from build123d import *

# Parameters (mm, degrees)
ESQUISSE1_R             = 25.4
BOSS_EXTRU_1_DEPTH      = 12.7
ESQUISSE2_R             = 1.3
ENL_V_MAT_EXTRU_1_DEPTH = 12.7


with BuildPart() as part:
    # Esquisse1 → Boss.-Extru.1 (new body)
    with BuildSketch(Plane.XY):
        Circle(ESQUISSE1_R)
    extrude(amount=BOSS_EXTRU_1_DEPTH)

    # Esquisse2 → Enlèv. mat.-Extru.1 (cut)
    with BuildSketch(Plane(origin=(0, 0, 0), x_dir=(-1, 0, 0), z_dir=(0, 0, -1))):
        Circle(ESQUISSE2_R)
        with Locations((0, 4.5)):
            Circle(ESQUISSE2_R)
        with Locations((0, 9)):
            Circle(ESQUISSE2_R)
        with Locations((0, 13.5)):
            Circle(ESQUISSE2_R)
        with Locations((0, 18)):
            Circle(ESQUISSE2_R)
        with Locations((3.897114317, 2.25)):
            Circle(ESQUISSE2_R)
        with Locations((3.897114317, -2.25)):
            Circle(ESQUISSE2_R)
        with Locations((0, -4.5)):
            Circle(ESQUISSE2_R)
        with Locations((-3.897114317, -2.25)):
            Circle(ESQUISSE2_R)
        with Locations((-3.897114317, 2.25)):
            Circle(ESQUISSE2_R)
        with Locations((4.5, 7.794228634)):
            Circle(ESQUISSE2_R)
        with Locations((7.794228634, 4.5)):
            Circle(ESQUISSE2_R)
        with Locations((9, 0)):
            Circle(ESQUISSE2_R)
        with Locations((7.794228634, -4.5)):
            Circle(ESQUISSE2_R)
        with Locations((4.5, -7.794228634)):
            Circle(ESQUISSE2_R)
        with Locations((0, -9)):
            Circle(ESQUISSE2_R)
        with Locations((-4.5, -7.794228634)):
            Circle(ESQUISSE2_R)
        with Locations((-7.794228634, -4.5)):
            Circle(ESQUISSE2_R)
        with Locations((-9, 0)):
            Circle(ESQUISSE2_R)
        with Locations((-7.794228634, 4.5)):
            Circle(ESQUISSE2_R)
        with Locations((-4.5, 7.794228634)):
            Circle(ESQUISSE2_R)
        with Locations((4.617271935, 12.685850381)):
            Circle(ESQUISSE2_R)
        with Locations((8.677632731, 10.341599982)):
            Circle(ESQUISSE2_R)
        with Locations((11.691342951, 6.75)):
            Circle(ESQUISSE2_R)
        with Locations((13.294904666, 2.344250399)):
            Circle(ESQUISSE2_R)
        with Locations((13.294904666, -2.344250399)):
            Circle(ESQUISSE2_R)
        with Locations((11.691342951, -6.75)):
            Circle(ESQUISSE2_R)
        with Locations((8.677632731, -10.341599982)):
            Circle(ESQUISSE2_R)
        with Locations((4.617271935, -12.685850381)):
            Circle(ESQUISSE2_R)
        with Locations((0, -13.5)):
            Circle(ESQUISSE2_R)
        with Locations((-4.617271935, -12.685850381)):
            Circle(ESQUISSE2_R)
        with Locations((-8.677632731, -10.341599982)):
            Circle(ESQUISSE2_R)
        with Locations((-11.691342951, -6.75)):
            Circle(ESQUISSE2_R)
        with Locations((-13.294904666, -2.344250399)):
            Circle(ESQUISSE2_R)
        with Locations((-13.294904666, 2.344250399)):
            Circle(ESQUISSE2_R)
        with Locations((-11.691342951, 6.75)):
            Circle(ESQUISSE2_R)
        with Locations((-8.677632731, 10.341599982)):
            Circle(ESQUISSE2_R)
        with Locations((-4.617271935, 12.685850381)):
            Circle(ESQUISSE2_R)
        with Locations((5.071186023, 17.270873525)):
            Circle(ESQUISSE2_R)
        with Locations((9.731534714, 15.142563591)):
            Circle(ESQUISSE2_R)
        with Locations((13.603492338, 11.787493211)):
            Circle(ESQUISSE2_R)
        with Locations((16.373375916, 7.477470234)):
            Circle(ESQUISSE2_R)
        with Locations((17.816785954, 2.561667089)):
            Circle(ESQUISSE2_R)
        with Locations((17.816785954, -2.561667089)):
            Circle(ESQUISSE2_R)
        with Locations((16.373375916, -7.477470234)):
            Circle(ESQUISSE2_R)
        with Locations((13.603492338, -11.787493211)):
            Circle(ESQUISSE2_R)
        with Locations((9.731534714, -15.142563591)):
            Circle(ESQUISSE2_R)
        with Locations((5.071186023, -17.270873525)):
            Circle(ESQUISSE2_R)
        with Locations((0, -18)):
            Circle(ESQUISSE2_R)
        with Locations((-5.071186023, -17.270873525)):
            Circle(ESQUISSE2_R)
        with Locations((-9.731534714, -15.142563591)):
            Circle(ESQUISSE2_R)
        with Locations((-13.603492338, -11.787493211)):
            Circle(ESQUISSE2_R)
        with Locations((-16.373375916, -7.477470234)):
            Circle(ESQUISSE2_R)
        with Locations((-17.816785954, -2.561667089)):
            Circle(ESQUISSE2_R)
        with Locations((-17.816785954, 2.561667089)):
            Circle(ESQUISSE2_R)
        with Locations((-16.373375916, 7.477470234)):
            Circle(ESQUISSE2_R)
        with Locations((-13.603492338, 11.787493211)):
            Circle(ESQUISSE2_R)
        with Locations((-9.731534714, 15.142563591)):
            Circle(ESQUISSE2_R)
        with Locations((-5.071186023, 17.270873525)):
            Circle(ESQUISSE2_R)
    extrude(amount=-ENL_V_MAT_EXTRU_1_DEPTH, mode=Mode.SUBTRACT)


solid = part.part
Read the model definition and answer for the solid it produces. Units are mm, in the model's axes. Round coordinates to 2 decimals unless told otherwise and drop trailing zeros. Loops run counter-clockwise (first coordinate to the right, second up) from the corner with the lowest first, then second, coordinate; pieces in that order, holes last.
Q1. Each of these flat-tipped pins is pushed along its axis until it touches: pin 1 (2 mm diameter, centred on x = 16.37, y = 7.48, fed in from +Z); pin 2 (5 mm diameter, centred on y = -8.5, z = 9, fed in from +X); pin 3 (2 mm diameter, centred on x = -7.5, z = 2, fed in from -Y). Where does it stop, or does it pass through?
Q2. Section B-B on y = 4.5 is taken. Write down the section's boundary in (x, z).
Q3. Section A-A on x = 14 is taken. Write down the section's boundary in (y, z), and give its area (3 significant figures).
Q4. Consider probe 1 along X at (y, z) = (17, 6); probe 2 along X at (y, z) = (-15.5, 11.75); probe 3 along Y at (x, z) = (-14, 11.75). Determine where each line is inside the solid, lowest interval first.
Q5. Section C-C on x = 0 is taken. Give the number of separate pieces and of enclosed holes in the cut face, and give its area (3 significant figures).
Output:
1. pin 1: passes through
1. pin 2: stops at x = 24.68
1. pin 3: stops at y = -24.55
2. outline: (-25, 0) - (-9.09, 0) - (-9.09, 12.7) - (-25, 12.7) - close; (-6.49, 0) - (-1.3, 0) - (-1.3, 12.7) - (-6.49, 12.7) - close; (1.3, 0) - (6.49, 0) - (6.49, 12.7) - (1.3, 12.7) - close; (9.09, 0) - (25, 0) - (25, 12.7) - (9.09, 12.7) - close
3. outline: (-21.19, 0) - (-13.03, 0) - (-13.03, 12.7) - (-21.19, 12.7) - close; (-10.55, 0) - (-3.44, 0) - (-3.44, 12.7) - (-10.55, 12.7) - close; (-1.25, 0) - (1.25, 0) - (1.25, 12.7) - (-1.25, 12.7) - close; (3.44, 0) - (10.55, 0) - (10.55, 12.7) - (3.44, 12.7) - close; (13.03, 0) - (21.19, 0) - (21.19, 12.7) - (13.03, 12.7) - close
3. area: 420 mm2
4. probe 1: x = -18.87 to -6.34, -3.8 to -0.83, 0.83 to 3.8, 6.34 to 18.87
4. probe 2: x = -20.12 to -10.98, -8.48 to 8.48, 10.98 to 20.12
4. probe 3: y = -21.19 to -13.03, -10.55 to -3.44, -1.25 to 1.25, 3.44 to 10.55, 13.03 to 21.19
5. separate pieces: 10
5. enclosed holes: 0
5. area: 348 mm2
